Design review of the part built by this model. Coordinates are the model's own, in mm. A direction names the side the tool comes from. Round coordinates to 2 decimals unless told otherwise and drop trailing zeros. Order: outer loops, then holes, each group sorted by start corner. A loop starts at its lowest first (then second) coordinate and runs counter-clockwise, first axis right, second up. Notation, with made-up numbers: M -31.5,33 L 6.5,33 A13 ccw 6.5,40 Z; hole C 81.25,-37.75 d9. An arc over 180 degrees is marked long. Use a Markdown table: item, result. Add a question column.
(1) Machinability: for faces 1 (the face through (-0.08, -0.63, -0.31)), 2 (the face through (-0.08, 0.63, 19.36)), 3 (the face through (0, 0, 19.685)), which of the approach directions +Z, -Z, +X, -X, +Y, -Y give a long, thin tool a straight path to every point of the face, cutting with its end or side? Answer none if there is none.
(2) For pin 1 (5.5 mm diameter, centred on x = 3.5, y = 3.5, fed in from +Z); pin 2 (5.5 mm diameter, centred on x = 4, y = 2, fed in from -Z), all flat-tipped, find the tip position at first contact; note any pin that passes through.
(3) Take a section at D-D (x = 3.25). Write out the cut boundary in (y, z) (3 decimals), then the cut area to 3 significant figures.
(4) Take a section at B-B (y = 0). Write out the cut boundary in (x, z) (3 decimals).
(5) To check wall thickness, follow probe 1 along Z at (x, y) = (5, -7.25); probe 2 along Y at (x, z) = (-8.25, 12) (3 decimals); probe 3 along X at (y, z) = (-8.5, 8) (3 decimals). State the ranges of each line that lie inside material, in increasing order. Write a range as from..to.
(6) Take a section at A-A (z = 6.75). Write out the cut boundary in (x, y) (3 decimals).
```python
from build123d import *

# Parameters (mm, degrees)
F0_W     = 19.05
F0_H     = 19.05
F1_DEPTH = 19.05
F2_R     = 0.635
F3_DEPTH = 0.635
F4_R     = 0.635
F5_DEPTH = 0.635
F6_SIZE  = 1.905


with BuildPart() as f1:
    # F0 (on Top) → F1 (new body)
    with BuildSketch(Plane.XY):
        Rectangle(F0_W, F0_H)
    extrude(amount=F1_DEPTH)

    # F2 (on face) → F3 (join)
    with BuildSketch(Plane.XY.offset(19.05)):
        Circle(F2_R)
    extrude(amount=F3_DEPTH)

    # F4 (on face) → F5 (join)
    with BuildSketch(Plane(origin=(0, 0, 0), x_dir=(1, 0, 0), z_dir=(0, 0, -1))):
        Circle(F4_R)
    extrude(amount=F5_DEPTH)

    # F6
    f6_edges = [f1.edges().sort_by_distance(p)[0] for p in [
        (-9.525, -9.525, 9.525),
        (9.525, -9.525, 9.525),
        (9.525, 9.525, 9.525),
        (-9.525, 9.525, 9.525),
    ]]
    chamfer(f6_edges, length=F6_SIZE)


solid = f1.part
```
Verdict:
| question | item | result |
|---|---|---|
| 1 | face 1 | -Z |
| 1 | face 2 | +Z |
| 1 | face 3 | +Z, +X, -X, +Y, -Y |
| 2 | pin 1 | stops at z = 19.05 |
| 2 | pin 2 | stops at z = 0 |
| 3 | outline | M -9.525,0 L 9.525,0 L 9.525,19.05 L -9.525,19.05 Z |
| 3 | area | 363 mm^2 |
| 4 | outline | M -9.525,0 L -0.635,0 L -0.635,-0.635 L 0.635,-0.635 L 0.635,0 L 9.525,0 L 9.525,19.05 L 0.635,19.05 L 0.635,19.685 L -0.635,19.685 L -0.635,19.05 L -9.525,19.05 Z |
| 5 | probe 1 | z = 0..19.05 |
| 5 | probe 2 | y = -8.895..8.895 |
| 5 | probe 3 | x = -8.645..8.645 |
| 6 | outline | M -9.525,-7.62 L -7.62,-9.525 L 7.62,-9.525 L 9.525,-7.62 L 9.525,7.62 L 7.62,9.525 L -7.62,9.525 L -9.525,7.62 Z |
